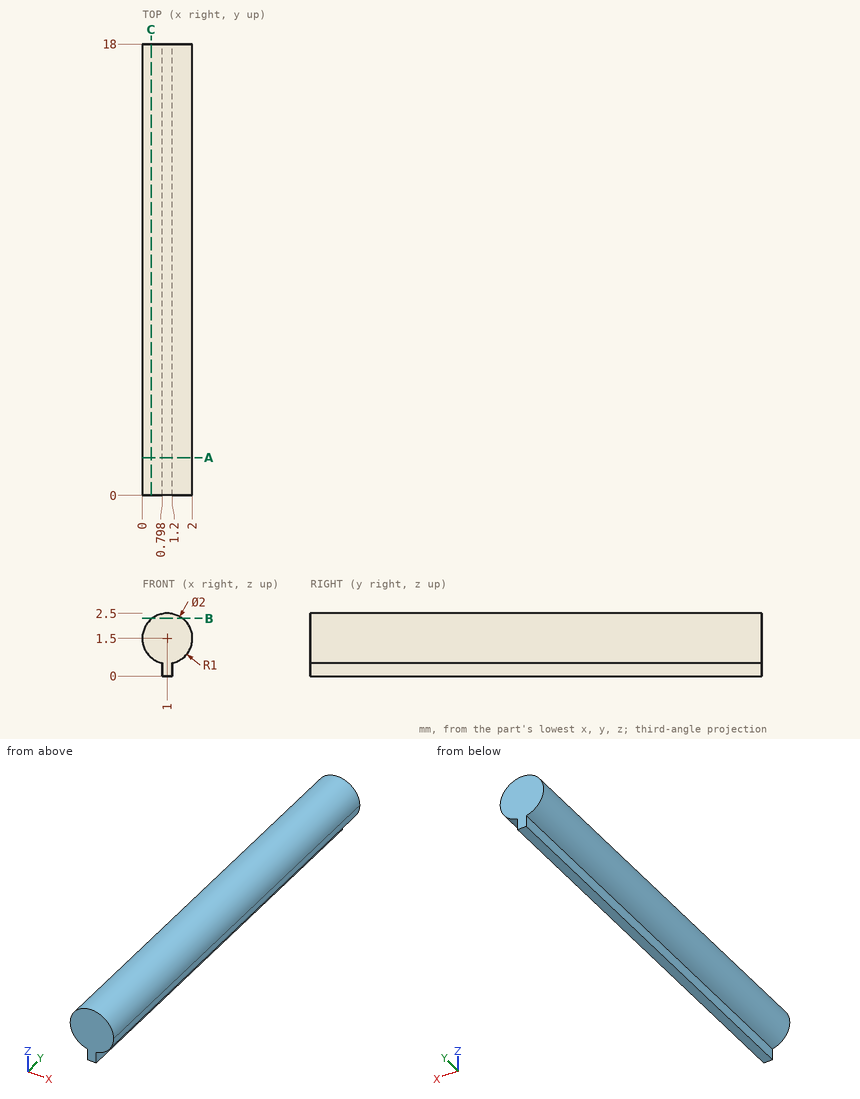
Part print with two shaded views. Sizes in mm from the minimum x, y, z corner. Give positions to 0.01 mm unless a question says otherwise; leave off trailing zeros. Order: outer loops, then holes, each group sorted by start corner. A loop starts at its lowest first (then second) coordinate and runs counter-clockwise, first axis right, second up.
(1) Saw through at B-B, the plane z = 2.3. Give the cut face in (x, y), then the cut area to 3 significant figures.
(2) Drill centre lines: L1, parallel to Z at x = 0.95, y = 17.25; L2, parallel to X at y = 13.75, z = 2.35 (1 decimal); L3, parallel to X at y = 15.25, z = 1.2 (1 decimal). Where is each one in solid material? Low to high.
(3) Flat gauge pin, fed straight in: pin 1 (1 mm diameter, centred on x = 1.5, y = 8.5, fed in from -Z). Where does the tip first touch, or does it go through?
(4) Saw through at A-A, the plane y = 1.5. Give the cut face in (x, z).
(5) Saw through at C-C, the plane x = 0.35. Give the cut face in (y, z).
Results found:
1. outline: (0.4, 0) - (1.6, 0) - (1.6, 18) - (0.4, 18) - close
1. area: 21.6 mm2
2. L1: z = 0 to 2.5
2. L2: x = 0.5 to 1.5
2. L3: x = 0 to 2
3. pin 1: stops at z = 0
4. outline: (0.8, 0) - (1.2, 0) - (1.2, 0.52) arc R1 ccw (long way) to (0.8, 0.52) - close
5. outline: (0, 0.74) - (18, 0.74) - (18, 2.26) - (0, 2.26) - close
